Input: part model. Units: mm. Frame: model coordinates. Face numbers are marked on the shaded views. A direction names the side the tool comes from. Round coordinates to 2 decimals unless told otherwise and drop trailing zeros. Order: outer loops, then holes, each group sorted by start corner. A loop starts at its lowest first (then second) coordinate and runs counter-clockwise, first axis right, second up. Notation, with made-up numbers: (-7, 3) -> (28, 3) arc R7 cw to (28, 14) -> close; hole circle Ø2 at (85.25, -11). An arc over 180 degrees is marked (long way). Use a Markdown table: item, result.
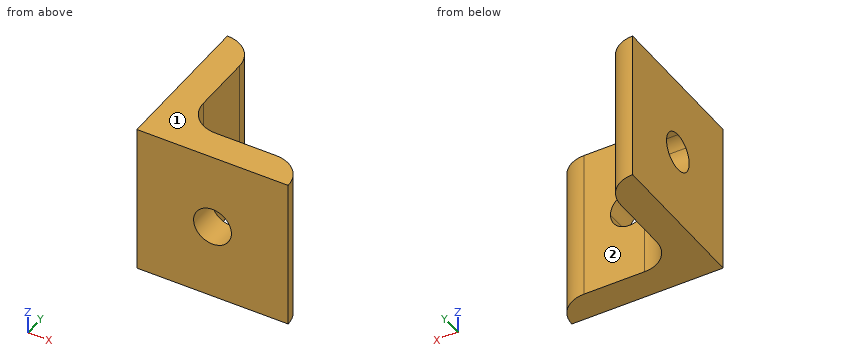
from build123d import *

# Parameters (mm, degrees)
BOSS_EXTRUDE1_DEPTH = 25.4
FILLET1_R           = 5.08
CUT_EXTRUDE1_DEPTH  = 25.4
CUT_EXTRUDE2_DEPTH  = 25.4


with BuildPart() as part:
    # Sketch1 → Boss-Extrude1 (new body)
    with BuildSketch(Plane.XY):
        Polygon((0, 0), (0, -25.4), (25.4, -25.4), (25.4, -20.32), (5.08, -20.32), (5.08, 0), align=None)
    extrude(amount=BOSS_EXTRUDE1_DEPTH)

    # Fillet1
    fillet1_edges = [part.edges().sort_by_distance(p)[0] for p in [
        (5.08, -20.32, 12.7),
        (5.08, 0, 12.7),
        (25.4, -20.32, 12.7),
    ]]
    fillet(fillet1_edges, radius=FILLET1_R - 0.0001)  # a hair under: the kernel refuses the full size

    # Sketch2 → Cut-Extrude1 (cut)
    with BuildSketch(Plane.XZ.offset(25.4)):
        with BuildLine():
            ThreePointArc((15.875, 12.7), (13.915019898, 15.633317516), (10.45493597, 14.94506403))
            Line((10.45493597, 14.94506403), (14.94506403, 10.45493597))
            ThreePointArc((14.94506403, 10.45493597), (15.633317516, 11.484980102), (15.875, 12.7))
        make_face()
        with BuildLine():
            Line((14.94506403, 10.45493597), (10.45493597, 14.94506403))
            ThreePointArc((10.45493597, 14.94506403), (10.45493597, 10.45493597), (14.94506403, 10.45493597))
        make_face()
    extrude(amount=-CUT_EXTRUDE1_DEPTH, mode=Mode.SUBTRACT)

    # Sketch3 → Cut-Extrude2 (cut)
    with BuildSketch(Plane.ZY):
        with BuildLine():
            ThreePointArc((10.45493597, -10.45493597), (10.45493597, -14.94506403), (14.94506403, -14.94506403))
            Line((14.94506403, -14.94506403), (10.45493597, -10.45493597))
        make_face()
        with BuildLine():
            Line((10.45493597, -10.45493597), (14.94506403, -14.94506403))
            ThreePointArc((14.94506403, -14.94506403), (15.633317516, -13.915019898), (15.875, -12.7))
            ThreePointArc((15.875, -12.7), (13.915019898, -9.766682484), (10.45493597, -10.45493597))
        make_face()
    extrude(amount=-CUT_EXTRUDE2_DEPTH, mode=Mode.SUBTRACT)


solid = part.part
1) Cut plane D-D on x = 17.5. Return loops of the section in (y, z).
Answer key:
| item | result |
|---|---|
| outline | (-25.4, 0) -> (-20.32, 0) -> (-20.32, 25.4) -> (-25.4, 25.4) -> close |
2) Cut plane A-A on x = 12.7. Return loops of the section in (y, z) (3 decimals), and give its area (3 significant figures).
Answer key:
| item | result |
|---|---|
| outline | (-25.4, 0) -> (-20.32, 0) -> (-20.32, 9.525) -> (-25.4, 9.525) -> close; (-25.4, 15.875) -> (-20.32, 15.875) -> (-20.32, 25.4) -> (-25.4, 25.4) -> close |
| area | 96.8 mm^2 |
3) Contact query for flat-ended pins moving along their axis: P1, Ø8, axis at y = -8.5, z = 11.5, coming from the +X side; P2, Ø1, axis at y = -11.5, z = 13, coming from the +X side; P3, Ø5, axis at x = 15.5, z = 18, coming from the +Y side. Output: stop coordinate, or through.
Answer key:
| item | result |
|---|---|
| P1 | stops at x = 5.08 |
| P2 | passes through |
| P3 | stops at y = -20.32 |
4) Ray query, probe 1 along X at (y, z) = (-6, 1.25); probe 2 along Y at (x, z) = (18, 5); probe 3 along Z at (x, y) = (3.75, -10). Return the intervals inside material, ascending.
Answer key:
| item | result |
|---|---|
| probe 1 | x = 0 to 5.08 |
| probe 2 | y = -25.4 to -20.32 |
| probe 3 | z = 0 to 11.03, 14.37 to 25.4 |
5) Set-up query: the marked faces 1 and 2. Return all of +Z, -Z, +X, -X, +Y, -Y with unobstructed straight access to the full face (end or side cutting, diameter ignored); none if empty.
Answer key:
| item | result |
|---|---|
| face 1 | +Z, +X, -X, +Y, -Y |
| face 2 | +Z, -Z, +X, +Y |
6) Cut plane C-C on z = 11.5. State how many separate pieces and enclosed holes the cut face has, and give its area (3 significant figures).
Answer key:
| item | result |
|---|---|
| separate pieces | 3 |
| enclosed holes | 0 |
| area | 167 mm^2 |
